```python
from build123d import *

# Parameters (mm, degrees)
PAD010_DEPTH    = 0.8
CHAMFER_SIZE    = 0.4
CHAMFER001_SIZE = 0.4
CHAMFER002_SIZE = 0.4
CHAMFER003_SIZE = 0.4


with BuildPart() as part:
    # Sketch018 → Pad010 (new body)
    with BuildSketch(Plane.XY):
        with BuildLine():
            Line((0, 1.5), (-4, 1.5))
            ThreePointArc((-4, 1.5), (-26.5, 4.148479), (-49, 1.5))
            ThreePointArc((-49, 1.5), (-50.055354, 0), (-49, -1.5))
            ThreePointArc((-49, -1.5), (-26.5, -4.148479), (-4, -1.5))
            Line((0, -1.5), (-4, -1.5))
            Line((0, 1.5), (0, -1.5))
        make_face()
    extrude(amount=PAD010_DEPTH)

    # Chamfer
    chamfer_edges = [part.edges().sort_by_distance(p)[0] for p in [
        (-2, 1.5, 0.8),
        (-2, -1.5, 0.8),
    ]]
    chamfer(chamfer_edges, length=CHAMFER_SIZE)

    # Chamfer001
    chamfer001_edges = [part.edges().sort_by_distance(p)[0] for p in [
        (-3.192094, 1.303463, 0.8),
        (-26.5, 4.148479, 0.8),
    ]]
    chamfer(chamfer001_edges, length=CHAMFER001_SIZE)

    # Chamfer002
    chamfer002_edges = [part.edges().sort_by_distance(p)[0] for p in [
        (-26.5, -4.148479, 0.8),
        (-3.192094, -1.303463, 0.8),
    ]]
    chamfer(chamfer002_edges, length=CHAMFER002_SIZE)

    # Chamfer003
    chamfer003_edges = [part.edges().sort_by_distance(p)[0] for p in [
        (-50.055354, 0, 0.8),
    ]]
    chamfer(chamfer003_edges, length=CHAMFER003_SIZE)


solid = part.part
```
The listing builds one solid part. Answer for the finished solid, in the listing's coordinates (mm). Coordinates: 2 decimals unless noted, no trailing zeros. Write each loop counter-clockwise with the first axis right and the second up, starting at its lowest first coordinate (ties: lowest second). Pieces come first, ordered by that corner, then holes. Notation, with made-up numbers: (-39, -15.75) - (-17, -15.75) arc R27 ccw to (-17, 5.25) - close; hole circle Ø1 at (-22, 34.25). An arc over 180 degrees is marked (long way). One line per item, written item: value.
1) This flat-tipped pin is pushed along its axis until it touches: pin 1 Ø4 at (x, y) = (-11, -1) entering from -Z. Where does it stop, or does it pass through?
Geometry check:
pin 1: stops at z = 0
2) Consider line 1 along Y through (x, z) = (-2.5, 0.4); line 2 along Y through (x, z) = (-20.5, 0.2); line 3 along X through (y, z) = (-0.5, 0.65). Determine where each line is inside the solid, lowest interval first. Write a range as from..to.
Geometry check:
line 1: y = -1.5..1.5
line 2: y = -3.96..3.96
line 3: x = -49.71..0
3) Find section A-A (z = 0.55). Give the vertices of the cut face in (x, y).
Geometry check:
outline: (-48.96, -1.36) arc R96.75 ccw to (-4.02, -1.35) - (0, -1.35) - (0, 1.35) - (-4.02, 1.35) arc R96.75 ccw to (-48.96, 1.36) arc R1.44 ccw to start
